Could you check a few things on this drawing? It's one solid part, dimensions in mm from its lowest x, y, z. Round coordinates to 2 decimals unless told otherwise and drop trailing zeros. Loops run counter-clockwise (first coordinate to the right, second up) from the corner with the lowest first, then second, coordinate; pieces in that order, holes last. Notation, with made-up numbers: M 15.25,47.25 L 69.25,47.25 A20 ccw 69.25,63.25 Z; hole C 13,-32.5 d1. An arc over 180 degrees is marked long. Put each result on its own line as item: value. Start each with the question number.
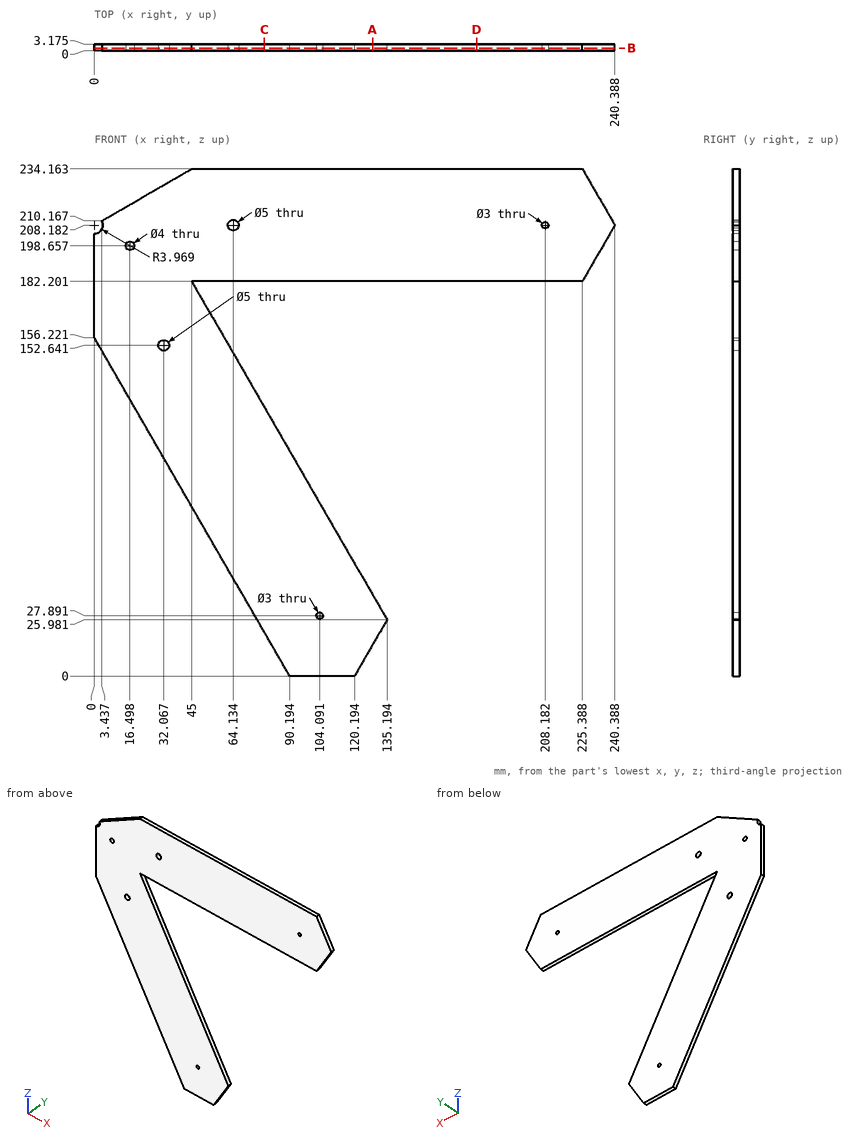
1) Suppose I cut it at D-D (x = 176.5). Write out the boundary of the cut face in (y, z) (1 decimal).
2) I'm going to push flat-ended pins straight in: P1, Ø1.5, axis at y = 0.5, z = 91.5, coming from the -X side; P2, Ø1.5, axis at y = 0.5, z = 78.5, coming from the +X side (1 decimal); P3, Ø1.5, axis at y = 2, z = 55.5, coming from the -X side. Where does each tip first touch, or does it pass through?
3) Suppose I cut it at A-A (x = 128.5). Write out the boundary of the cut face in (y, z) (1 decimal).
4) If I drill on probe 1 along X at (y, z) = (2.35, 208) (1 decimal); probe 2 along Z at (x, y) = (211, 2.3); probe 3 along Z at (x, y) = (115, 1.2) (1 decimal), over which ranges is the centre line in solid material (lowest first)? Write a range as from..to.
5) Suppose I cut it at B-B (y = 1.25). Write out the boundary of the cut face in (x, z) (1 decimal), plus the area to 3 significant figures.
6) Suppose I cut it at C-C (x = 78.5). Write out the boundary of the cut face in (y, z) (1 decimal), plus the area to 3 significant figures.
Results are:
1. outline: M 0,182.2 L 3.2,182.2 L 3.2,234.2 L 0,234.2 Z
2. P1: x = 36.93
2. P2: x = 105.3
2. P3: x = 57.72
3. outline: M 0,14.4 L 3.2,14.4 L 3.2,37.6 L 0,37.6 Z; M 0,182.2 L 3.2,182.2 L 3.2,234.2 L 0,234.2 Z
4. probe 1: 4..61.6, 66.6..206.7, 209.7..240.3
4. probe 2: 182.2..234.16
4. probe 3: 0..61, 182.2..234.2
5. outline: M 0,156.2 L 90.2,0 L 120.2,0 L 135.2,26 L 45,182.2 L 225.4,182.2 L 240.4,208.2 L 225.4,234.2 L 45,234.2 L 3.4,210.2 A4 cw 0,204.2 Z; hole C 16.5,198.7 d4; hole C 32.1,152.6 d5; hole C 64.1,208.2 d5; hole C 104.1,27.9 d3; hole C 208.2,208.2 d3
5. area: 21,800 mm²
6. outline: M 0,20.3 L 3.2,20.3 L 3.2,124.2 L 0,124.2 Z; M 0,182.2 L 3.2,182.2 L 3.2,234.2 L 0,234.2 Z
6. area: 495 mm²
